Model file for the job. Use its own axes, mm. A direction names the side the tool comes from. Give positions to 0.01 mm unless a question says otherwise; leave off trailing zeros. Write each loop counter-clockwise with the first axis right and the second up, starting at its lowest first coordinate (ties: lowest second). Pieces come first, ordered by that corner, then holes. Notation, with made-up numbers: (3, 77.25) - (27, 77.25) arc R24 ccw to (27, 100.25) - close; hole circle Ø9 at (-10, -28). An arc over 180 degrees is marked (long way). Use CSV: the item, a comma, the result in double quotes.
from build123d import *

# Parameters (mm, degrees)
F0_W     = 450
F0_H     = 450
F0_R     = 10
F1_DEPTH = 40
F2_R     = 10
F3_DEPTH = 80


# Not quite as in the source:
# - the program builds the solid bodies; features that only make, move or delete a surface that nothing else refers to are left out


with BuildPart() as f1:
    # F0 (on Top) → F1 (new body)
    with BuildSketch(Plane.XY):
        Rectangle(F0_W, F0_H)
        with Locations((-200, -200)):
            Circle(F0_R, mode=Mode.SUBTRACT)
        with Locations((200, -200)):
            Circle(F0_R, mode=Mode.SUBTRACT)
        with Locations((-200, 200)):
            Circle(F0_R, mode=Mode.SUBTRACT)
        with Locations((200, 200)):
            Circle(F0_R, mode=Mode.SUBTRACT)
    extrude(amount=F1_DEPTH)

    # F2 (on face) → F3 (join)
    with BuildSketch(Plane.XY.offset(40)):
        with Locations((-200, -200)):
            Circle(F2_R)
    extrude(amount=-F3_DEPTH)


solid = f1.part
(1) Flat gauge pins, fed straight in: P1, Ø6, axis at x = -40.5, y = 169, coming from the -Z side; P2, Ø18, axis at x = 200, y = 200, coming from the +Z side. Where does each tip first touch, or does it go through?
Checked values:
P1,"stops at z = 0"
P2,"passes through"
(2) Saw through at A-A, the plane x = -200. List the corners of the cut face in (y, z), then the cut area to 3 significant figures.
Checked values:
outline,"(-225, 0) - (-210, 0) - (-210, -40) - (-190, -40) - (-190, 0) - (190, 0) - (190, 40) - (-225, 40) - close; (210, 0) - (225, 0) - (225, 40) - (210, 40) - close"
area,"18,000 mm^2"
(3) Saw through at D-D, the plane z = -31. List the corners of the cut face in (x, y).
Checked values:
outline,"circle Ø20 at (-200, -200)"
(4) Pull direction X, two halves, no side cores. Call faces 3 (the face through (225, -3, 20)), 4 (the face through (-190.763, 196.17, 19.72)), 5 (the face through (209.237, 196.17, 19.72)), 6 (the face through (-3, 3, 0)): released by +X, released by -X, zero draft, split by the parting line, or undercut.
Checked values:
face 3,"released by +X"
face 4,"undercut"
face 5,"undercut"
face 6,"zero draft"
(5) Wall check: probe 1 along Y at (x, z) = (200, 11); probe 2 along Y at (x, z) = (-200, 17); probe 3 along Z at (x, y) = (108.5, -188). Give the ranges that are in metal, low to high. Write a range as [from, to].
Checked values:
probe 1,"y = [-225, -210], [-190, 190], [210, 225]"
probe 2,"y = [-225, 190], [210, 225]"
probe 3,"z = [0, 40]"
(6) 3-axis set-ups, long thin cutter, end or side, ignore diameter. For faces 1 (the face through (-225, -3, 20)), 2 (the face through (-190.763, -203.83, -19.72)): which of +Z, -Z, +X, -X, +Y, -Y reach the whole face in a straight line?
Checked values:
face 1,"+Z, -Z, -X, +Y, -Y"
face 2,"-Z"
(7) Saw through at C-C, the plane x = 200. List the corners of the cut face in (y, z).
Checked values:
outline,"(-225, 0) - (-210, 0) - (-210, 40) - (-225, 40) - close; (-190, 0) - (190, 0) - (190, 40) - (-190, 40) - close; (210, 0) - (225, 0) - (225, 40) - (210, 40) - close"
